Could you check a few things on this drawing? It's one solid part, dimensions in mm from its lowest x, y, z. A direction names the side the tool comes from. Coordinates: 2 decimals unless noted, no trailing zeros. Order: outer loops, then holes, each group sorted by start corner. A loop starts at its lowest first (then second) coordinate and runs counter-clockwise, first axis right, second up. Notation, with made-up numbers: M -3,43 L 4,43 A24 ccw 4,58 Z; hole C -30,3.5 d5. An arc over 180 degrees is marked long. Write item = value, one per line. Start each with the question number.
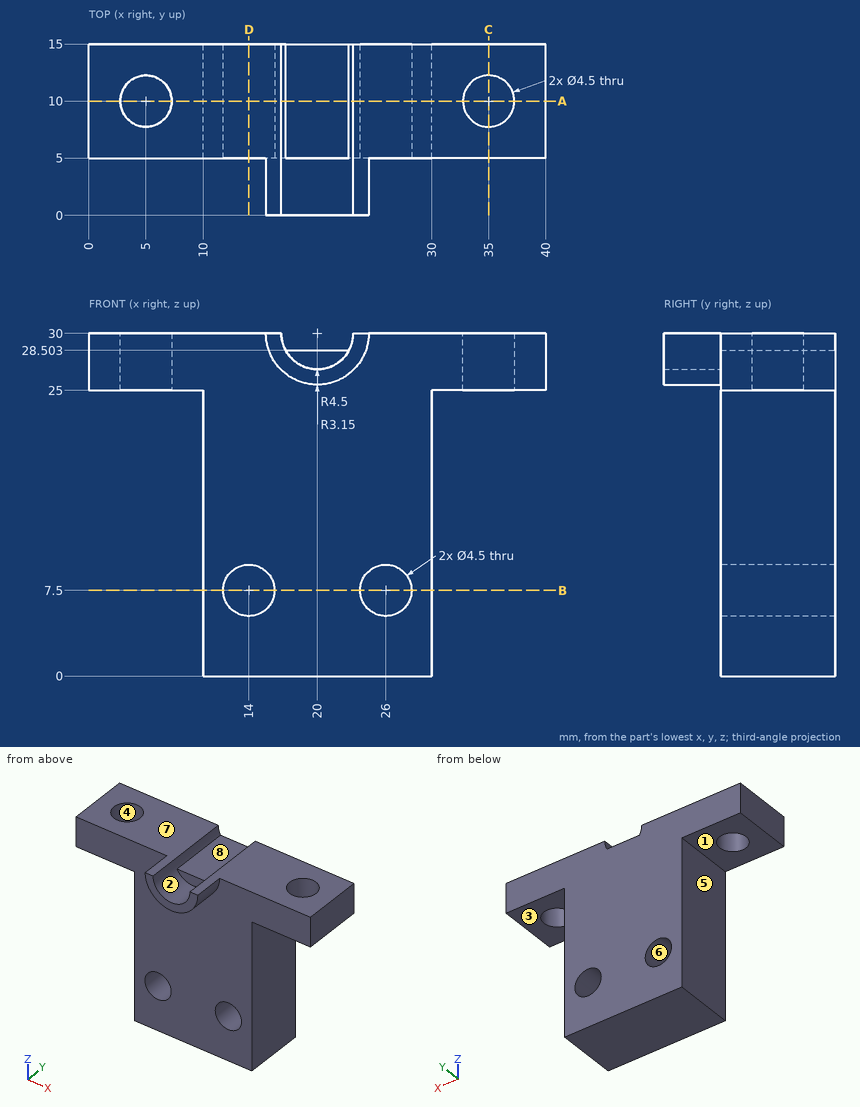
(1) Imagine slicing it at D-D on x = 14. List the corners of the cut face in (y, z) for me, plus the area to 3 significant figures.
(2) Imagine slicing it at A-A on y = 10. List the corners of the cut face in (x, z) for me, plus the area to 3 significant figures.
(3) Will these pins go through, and if not, where does the flat tip stop? P1, Ø8, axis at y = 10, z = 14, coming from the +X side; P2, Ø3, axis at x = 33.5, z = 22.5, coming from the +Y side; P3, Ø5, axis at x = 14, z = 25, coming from the -Y side; P4, Ø3, axis at y = 11.5, z = 12.5, coming from the -X side.
(4) Thinking about a two-plate mould opening in X: for the marked faces 5, 6, 7 and 8, which applies, released by +X, released by -X, zero draft, split by the parting line, or undercut?
(5) Imagine slicing it at C-C on x = 35. List the corners of the cut face in (y, z) for me, plus the area to 3 significant figures.
(6) Imagine slicing it at B-B on z = 7.5. List the corners of the cut face in (x, y) for me, plus the area to 3 significant figures.
(7) For the marked faces 1, 2, 3 and 4, which set-ups out of +Z, -Z, +X, -X, +Y, -Y let a thin tool reach every point of the face, with its end or its side?
(8) Please list where these lines run through material, in increasing order: probe 1 along Z at (x, y) = (26, 11.75); probe 2 along Y at (x, z) = (5, 26.75); probe 3 along X at (y, z) = (11.75, 8) (1 decimal). Write a range as from..to.
Response:
q1.outline = M 5,0 L 15,0 L 15,5.25 L 5,5.25 Z; M 5,9.75 L 15,9.75 L 15,30 L 5,30 Z
q1.area = 255 mm2
q2.outline = M 0,25 L 2.75,25 L 2.75,30 L 0,30 Z; M 7.25,25 L 10,25 L 10,0 L 30,0 L 30,25 L 32.75,25 L 32.75,30 L 23.15,30 A3.15 cw 22.77,28.5 L 17.23,28.5 A3.15 cw 16.85,30 L 7.25,30 Z; M 37.25,25 L 40,25 L 40,30 L 37.25,30 Z; hole C 14,7.5 d4.5; hole C 26,7.5 d4.5
q2.area = 614 mm2
q3.P1 = 30
q3.P2 = through
q3.P3 = 5
q3.P4 = 10
q4.face_5 = released by -X
q4.face_6 = undercut
q4.face_7 = zero draft
q4.face_8 = undercut
q5.outline = M 5,25 L 7.75,25 L 7.75,30 L 5,30 Z; M 12.25,25 L 15,25 L 15,30 L 12.25,30 Z
q5.area = 27.5 mm2
q6.outline = M 10,5 L 11.75,5 L 11.75,15 L 10,15 Z; M 16.25,5 L 23.75,5 L 23.75,15 L 16.25,15 Z; M 28.25,5 L 30,5 L 30,15 L 28.25,15 Z
q6.area = 110 mm2
q7.face_1 = -Z, -X, +Y, -Y
q7.face_2 = +Z, -Y
q7.face_3 = -Z, +X, +Y, -Y
q7.face_4 = +Z, -Z
q8.probe_1 = 0..5.25, 9.75..30
q8.probe_2 = 5..7.75, 12.25..15
q8.probe_3 = 10..11.8, 16.2..23.8, 28.2..30
